from build123d import *

# Parameters (mm, degrees)
SKETCH_1_R      = 1.5
EXTRUDE_1_DEPTH = 5


with BuildPart() as part:
    # 스케치1 → 보스-돌출1 (new body)
    with BuildSketch(Plane(origin=(0, 0, 0), x_dir=(1, 0, 0), z_dir=(0, 1, 0))):
        Polygon((59.481067557, -143.6), (143.6, -59.481067557), (143.6, 59.481067557), (59.481067557, 143.6), (-59.481067557, 143.6), (-143.6, 59.481067557), (-143.6, -59.481067557), (-59.481067557, -143.6), align=None)
        with Locations((-5, 138.54)):
            Circle(SKETCH_1_R, mode=Mode.SUBTRACT)
        with Locations((-5, 128.54)):
            Circle(SKETCH_1_R, mode=Mode.SUBTRACT)
        with Locations((5, 128.54)):
            Circle(SKETCH_1_R, mode=Mode.SUBTRACT)
        with Locations((5, 138.54)):
            Circle(SKETCH_1_R, mode=Mode.SUBTRACT)
        with Locations((138.54, 5)):
            Circle(SKETCH_1_R, mode=Mode.SUBTRACT)
        with Locations((128.54, 5)):
            Circle(SKETCH_1_R, mode=Mode.SUBTRACT)
        with Locations((128.54, -5)):
            Circle(SKETCH_1_R, mode=Mode.SUBTRACT)
        with Locations((138.54, -5)):
            Circle(SKETCH_1_R, mode=Mode.SUBTRACT)
        with Locations((5, -138.54)):
            Circle(SKETCH_1_R, mode=Mode.SUBTRACT)
        with Locations((5, -128.54)):
            Circle(SKETCH_1_R, mode=Mode.SUBTRACT)
        with Locations((-5, -128.54)):
            Circle(SKETCH_1_R, mode=Mode.SUBTRACT)
        with Locations((-5, -138.54)):
            Circle(SKETCH_1_R, mode=Mode.SUBTRACT)
        with Locations((-138.54, -5)):
            Circle(SKETCH_1_R, mode=Mode.SUBTRACT)
        with Locations((-128.54, -5)):
            Circle(SKETCH_1_R, mode=Mode.SUBTRACT)
        with Locations((-128.54, 5)):
            Circle(SKETCH_1_R, mode=Mode.SUBTRACT)
        with Locations((-138.54, 5)):
            Circle(SKETCH_1_R, mode=Mode.SUBTRACT)
    extrude(amount=EXTRUDE_1_DEPTH)


solid = part.part
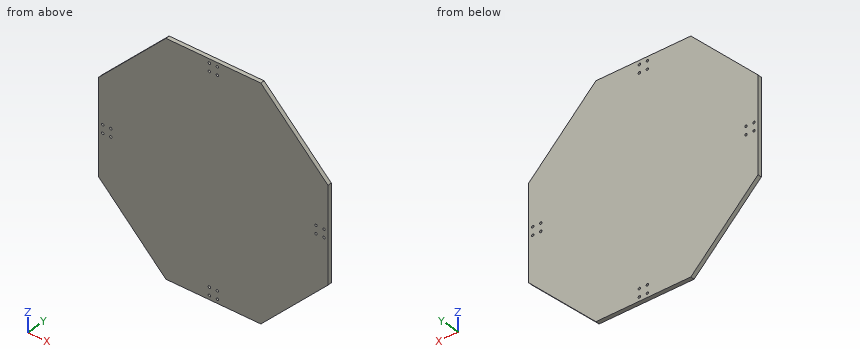
Geometry check sheet. Reference: the model listing, model coordinates, mm. Round coordinates to 2 decimals unless told otherwise and drop trailing zeros. Order: outer loops, then holes, each group sorted by start corner. A loop starts at its lowest first (then second) coordinate and runs counter-clockwise, first axis right, second up. Notation, with made-up numbers: M 80,26.5 L 100,26.5 A19 ccw 100,61.5 Z; hole C 83.25,51 d4. An arc over 180 degrees is marked long. Answer in a Markdown table with one row per item. Add a question column.
Item 1: Material ranges on L1, parallel to X at y = 1.95, z = -5; L2, parallel to X at y = 1.5, z = -128.54, recorded low to high. Write a range as [from, to].
Item 2: Depth check by flat-ended pin: pin 1 Ø1.8 at (x, z) = (128.54, 5) entering from +Y (3 decimals); pin 2 Ø2 at (x, y) = (104, 4) entering from -Z; pin 3 Ø1.5 at (x, y) = (112.5, 1.5) entering from -Z. Enter the tip coordinate at first touch or a pass-through.
Item 3: Sectioned sample at B-B, the plane z = -82. Enter the section's corners in (x, y).
Item 4: Sectioned sample at C-C, the plane x = -108. Enter the section's corners in (y, z), plus the area to 3 significant figures.
Item 5: Sectioned sample at A-A, the plane y = 2.45. State how many separate pieces and enclosed holes the cut face has, plus the area to 3 significant figures.
Filled in:
| question | item | result |
|---|---|---|
| 1 | L1 | x = [-143.6, -140.04], [-137.04, -130.04], [-127.04, 127.04], [130.04, 137.04], [140.04, 143.6] |
| 1 | L2 | x = [-74.54, -6.5], [-3.5, 3.5], [6.5, 74.54] |
| 2 | pin 1 | passes through |
| 2 | pin 2 | stops at z = -100.08 |
| 2 | pin 3 | stops at z = -91.33 |
| 3 | outline | M -121.08,0 L 121.08,0 L 121.08,5 L -121.08,5 Z |
| 4 | outline | M 0,-95.08 L 5,-95.08 L 5,95.08 L 0,95.08 Z |
| 4 | area | 951 mm² |
| 5 | separate pieces | 1 |
| 5 | enclosed holes | 16 |
| 5 | area | 68,200 mm² |
